Check sheet for the modelled part. Datum: model origin and axes. Units: mm. A direction names the side the tool comes from. Give positions to 0.01 mm unless a question says otherwise; leave off trailing zeros. Loops run counter-clockwise (first coordinate to the right, second up) from the corner with the lowest first, then second, coordinate; pieces in that order, holes last. Notation, with made-up numbers: M 18,61.5 L 36,61.5 A16 cw 36,67.5 Z; hole C 78.25,13.5 d5. An arc over 180 degrees is marked long. Use one line per item in the form item = value.
from build123d import *

# Parameters (mm, degrees)
ESBO_O1_R                = 2.5
RESSALTO_EXTRUS_O1_DEPTH = 75
FILETE1_R                = 2


with BuildPart() as part:
    # Esboço1 → Ressalto-extrusão1 (new, symmetric)
    with BuildSketch(Plane(origin=(0, 0, 0), x_dir=(0, 0, -1), z_dir=(1, 0, 0))):
        with BuildLine():
            Line((-100, -17.848056111), (0, -19.347346796))
            Line((0, -19.347346796), (116.020534247, -0.683058506))
            Line((116.020534247, -0.683058506), (42.496745606, -0.683058506))
            Line((42.496745606, -0.683058506), (-15.006508788, 19.480520471))
            ThreePointArc((-15.006508788, 19.480520471), (-16.311915051, 27.040473041), (-22.459012532, 22.450248543))
            Line((-22.459012532, 22.450248543), (-97.460720141, 21.975419182))
            ThreePointArc((-97.460720141, 21.975419182), (-104.830140039, 25.877112836), (-102.267981422, 17.941943889))
            Line((-102.267981422, 17.941943889), (-100, -17.848056111))
        make_face()
        with Locations((-101.937720305, 22.42980837)):
            Circle(ESBO_O1_R, mode=Mode.SUBTRACT)
        with Locations((-17.977720305, 22.860150942)):
            Circle(ESBO_O1_R, mode=Mode.SUBTRACT)
    extrude(amount=RESSALTO_EXTRUS_O1_DEPTH, both=True)

    # Filete1
    filete1_edges = [part.edges().sort_by_distance(p)[0] for p in [
        (0, -0.683058506, -116.020534247),
    ]]
    fillet(filete1_edges, radius=FILETE1_R)


solid = part.part
1) Section check A-A (x = -4.5). Record the cut outline in (y, z), then the cut area to 3 significant figures.
Evaluation:
outline = M -19.35,0 L -4.66,-91.31 A2 ccw -0.68,-91 L -0.68,-42.5 L 19.48,15.01 A4.5 ccw long 22.45,22.46 L 21.98,97.46 A4.5 ccw long 17.94,102.27 L -17.85,100 Z; hole C 22.43,101.94 d5; hole C 22.86,17.98 d5
area = 5,450 mm^2
2) Depth check by flat-ended pin: pin 1 Ø3 at (x, z) = (-49, 82.5) entering from -Y; pin 2 Ø4 at (x, z) = (41.5, -55.5) entering from -Y; pin 3 Ø3 at (x, z) = (-54, 32.5) entering from -Y; pin 4 Ø3 at (y, z) = (22.43, 101.94) entering from -X. Enter the tip coordinate at first touch or a pass-through.
Evaluation:
pin_1 = -18.13
pin_2 = -10.74
pin_3 = -18.88
pin_4 = through
3) Scan lines: line 1 (Z direction, x = 33.5, y = 22.5); line 2 (Z direction, x = 50, y = 21); line 3 (Z direction, x = 65.5, y = 23). Record each from-to range of solid material in increasing order.
Evaluation:
line_1 = 13.49 to 15.5, 20.45 to 22.46, 97.44 to 99.44, 104.44 to 106.44
line_2 = 13.88 to 16.31, 19.65 to 99.89, 103.99 to 106.2
line_3 = 13.48 to 15.48, 20.47 to 22.48, 97.47 to 99.5, 104.37 to 106.4
4) Section check B-B (z = 73). Record the cut outline in (x, y).
Evaluation:
outline = M -75,-18.25 L 75,-18.25 L 75,22.13 L -75,22.13 Z
5) Release check for a two-part mould opening along Z. For faces 1 (the face through (1.05, 25.971, 104.714)), 2 (the face through (-75, -1, 30)), 3 (the face through (1.05, -12.105, -45.018)) record: pulls with the +Z half, pulls with the -Z half, needs draft (parallel to the pull), parting line crosses it, or undercut.
Evaluation:
face_1 = undercut
face_2 = needs draft
face_3 = pulls with the -Z half
6) Section check C-C (y = 4). Record the cut outline in (x, z).
Evaluation:
outline = M -75,-29.14 L 75,-29.14 L 75,101.38 L -75,101.38 Z
7) Set-up check for faces 4 (the face through (1, -0.683, -67)), 5 (the face through (-1.05, 21.47, 99.63)): record each of +Z, -Z, +X, -X, +Y, -Y from which the full face is reachable in a straight line by a thin tool's end or side.
Evaluation:
face_4 = -Z, +X, -X, +Y
face_5 = +X, -X
